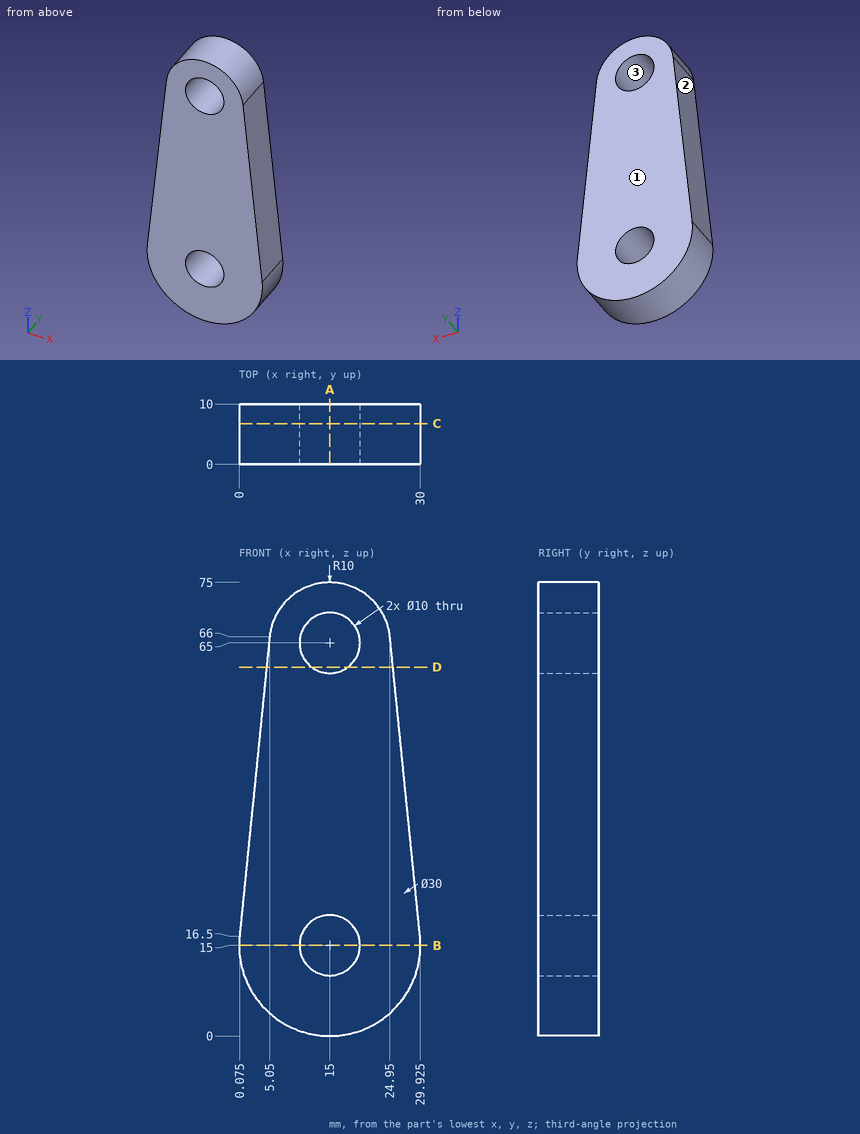
Could you check a few things on this drawing? It's one solid part, dimensions in mm from its lowest x, y, z. Coordinates: 2 decimals unless noted, no trailing zeros. Write each loop counter-clockwise with the first axis right and the second up, starting at its lowest first coordinate (ties: lowest second). Pieces come first, ordered by that corner, then holes.
Q1. If we mould it in two halves opening along Z, with no side actions, what happens to the marked faces 1, 2 and 3? For each: +Z half, -Z half, draft (parallel to the pull), parting line (faces both ways), or undercut.
Results found:
face 1: draft
face 2: +Z half
face 3: undercut
Q2. Please list where these lines run through material, in increasing order: L1, parallel to Z at x = 15, y = 5.5; L2, parallel to Z at x = 11, y = 4.75 (1 decimal); L3, parallel to X at y = 7.25, z = 64.
Results found:
L1: z = 0 to 10, 20 to 60, 70 to 75
L2: z = 0.5 to 12, 18 to 62, 68 to 74.2
L3: x = 4.85 to 10.1, 19.9 to 25.15
Q3. Imagine slicing it at D-D, the plane z = 61. List the corners of the cut face in (x, y) for me.
Results found:
outline: (4.55, 0) - (12, 0) - (12, 10) - (4.55, 10) - close; (18, 0) - (25.45, 0) - (25.45, 10) - (18, 10) - close
Q4. Imagine slicing it at A-A, the plane x = 15. List the corners of the cut face in (y, z) for me, plus the area to 3 significant figures.
Results found:
outline: (0, 0) - (10, 0) - (10, 10) - (0, 10) - close; (0, 20) - (10, 20) - (10, 60) - (0, 60) - close; (0, 70) - (10, 70) - (10, 75) - (0, 75) - close
area: 550 mm2
Q5. Imagine slicing it at B-B, the plane z = 15. List the corners of the cut face in (x, y) for me.
Results found:
outline: (0, 0) - (10, 0) - (10, 10) - (0, 10) - close; (20, 0) - (30, 0) - (30, 10) - (20, 10) - close
Q6. For P1, Ø13, axis at x = 15, z = 15, coming from the -Y side; P2, Ø3, axis at x = 7.5, y = 2.5, coming from the -Z side; P3, Ø6, axis at y = 4, z = 55.5, coming from the +X side; P4, Ø1.5, axis at y = 1.5, z = 63, coming from the +X side, each with a flat end and sliding along its axis, tell me the tip position at first contact or that it passes through.
Results found:
P1: stops at y = 0
P2: stops at z = 1.25
P3: stops at x = 26.31
P4: stops at x = 25.33
Q7. Imagine slicing it at C-C, the plane y = 6.75. Count the separate pieces of the cut face and the enclosed holes in it, plus the area to 3 significant figures.
Results found:
separate pieces: 1
enclosed holes: 2
area: 1,610 mm2
